CAD build for the part. Positions are in the model's coordinates, mm. Face numbers are marked on the shaded views. A direction names the side the tool comes from. Give positions to 0.01 mm unless a question says otherwise; leave off trailing zeros. Write each loop counter-clockwise with the first axis right and the second up, starting at its lowest first coordinate (ties: lowest second). Pieces come first, ordered by that corner, then holes. Notation, with made-up numbers: (-5.5, 46) - (26.5, 46) arc R21 cw to (26.5, 64) - close; hole circle Ø10 at (71.5, 51). An arc over 180 degrees is marked (long way). Answer as a JSON object with one key per item and string values.
from build123d import *

# Parameters (mm, degrees)
EXTRUDE_1_DEPTH     = 15.1
EXTRUDE_START       = -3.88
EXTRUDE_2_DEPTH     = 3.88
CUT_EXTRUDE_1_REACH = 37.992


with BuildPart() as part:
    # 草图1 → 凸台-拉伸1 (new body)
    with BuildSketch(Plane.XY):
        with BuildLine():
            Line((-15.4, 3.2), (-15.4, 7.25))
            ThreePointArc((-15.4, 7.25), (-14.330939751, 9.830939751), (-11.75, 10.9))
            Line((-11.75, 10.9), (11.75, 10.9))
            ThreePointArc((11.75, 10.9), (14.330939751, 9.830939751), (15.4, 7.25))
            Line((15.4, 7.25), (15.4, -7.25))
            ThreePointArc((15.4, -7.25), (14.330939751, -9.830939751), (11.75, -10.9))
            Line((11.75, -10.9), (3.85, -10.9))
            Line((3.85, -10.9), (-3.85, -10.9))
            Line((-3.85, -10.9), (-11.75, -10.9))
            ThreePointArc((-11.75, -10.9), (-14.330939751, -9.830939751), (-15.4, -7.25))
            Line((-15.4, -7.25), (-15.4, 3.2))
        make_face()
        with BuildLine():
            Line((-13.4, 3.2), (-13.4, 7.25))
            ThreePointArc((-13.4, 7.25), (-12.916726189, 8.416726189), (-11.75, 8.9))
            Line((-11.75, 8.9), (11.75, 8.9))
            ThreePointArc((11.75, 8.9), (12.916726189, 8.416726189), (13.4, 7.25))
            Line((13.4, 7.25), (13.4, -7.25))
            ThreePointArc((13.4, -7.25), (12.916726189, -8.416726189), (11.75, -8.9))
            Line((11.75, -8.9), (3.85, -8.9))
            Line((3.85, -8.9), (-3.85, -8.9))
            Line((-3.85, -8.9), (-11.75, -8.9))
            ThreePointArc((-11.75, -8.9), (-12.916726189, -8.416726189), (-13.4, -7.25))
            Line((-13.4, -7.25), (-13.4, 3.2))
        make_face(mode=Mode.SUBTRACT)
    extrude(amount=-EXTRUDE_1_DEPTH)

    # 草图2 → 凸台-拉伸2 (add)
    with BuildSketch(Plane(origin=(0, 0, -15.1), x_dir=(-1, 0, 0), z_dir=(0, 0, -1)).offset(EXTRUDE_START)):
        with BuildLine():
            Line((-13.4, 6.82), (-13.25, 6.82))
            Line((-13.25, 6.82), (-11.67, 6.82))
            ThreePointArc((-11.67, 6.82), (-11.422512627, 6.922512627), (-11.32, 7.17))
            Line((-11.32, 7.17), (-11.32, 8.75))
            Line((-11.32, 8.75), (-11.32, 8.9))
            Line((-11.32, 8.9), (-11.75, 8.9))
            ThreePointArc((-11.75, 8.9), (-12.916726189, 8.416726189), (-13.4, 7.25))
            Line((-13.4, 7.25), (-13.4, 6.82))
        make_face()
        with BuildLine():
            Line((-13.25, -5.02), (-13.4, -5.02))
            Line((-13.4, -5.02), (-13.4, -7.25))
            ThreePointArc((-13.4, -7.25), (-12.916726189, -8.416726189), (-11.75, -8.9))
            Line((-11.75, -8.9), (-9.52, -8.9))
            Line((-9.52, -8.9), (-9.52, -8.75))
            Line((-9.52, -8.75), (-9.52, -5.87))
            ThreePointArc((-9.52, -5.87), (-9.768959236, -5.268959236), (-10.37, -5.02))
            Line((-10.37, -5.02), (-13.25, -5.02))
        make_face()
        with BuildLine():
            Line((9.52, -8.75), (9.52, -8.9))
            Line((9.52, -8.9), (11.75, -8.9))
            ThreePointArc((11.75, -8.9), (12.916726189, -8.416726189), (13.4, -7.25))
            Line((13.4, -7.25), (13.4, -5.02))
            Line((13.4, -5.02), (13.25, -5.02))
            Line((13.25, -5.02), (10.37, -5.02))
            ThreePointArc((10.37, -5.02), (9.768959236, -5.268959236), (9.52, -5.87))
            Line((9.52, -5.87), (9.52, -8.75))
        make_face()
        with BuildLine():
            Line((11.75, 8.9), (11.32, 8.9))
            Line((11.32, 8.9), (11.32, 8.75))
            Line((11.32, 8.75), (11.32, 7.17))
            ThreePointArc((11.32, 7.17), (11.422512627, 6.922512627), (11.67, 6.82))
            Line((11.67, 6.82), (13.25, 6.82))
            Line((13.25, 6.82), (13.4, 6.82))
            Line((13.4, 6.82), (13.4, 7.25))
            ThreePointArc((13.4, 7.25), (12.916726189, 8.416726189), (11.75, 8.9))
        make_face()
    extrude(amount=EXTRUDE_2_DEPTH)

    # 草图3 → 切除-拉伸1 (cut, up to next)
    with BuildSketch(Plane.ZY.offset(15.4), mode=Mode.PRIVATE) as cut_extrude_1_sk1:
        with BuildLine():
            Line((0.15, 8.9), (-4, 8.9))
            ThreePointArc((-4, 8.9), (-4.247487373, 8.797487373), (-4.35, 8.55))
            Line((-4.35, 8.55), (-4.35, 3.55))
            ThreePointArc((-4.35, 3.55), (-4.247487373, 3.302512627), (-4, 3.2))
            Line((-4, 3.2), (0.15, 3.2))
            Line((0.15, 3.2), (0.15, 8.9))
        make_face()
    cut_extrude_1_tool1 = extrude(cut_extrude_1_sk1.sketch, amount=-CUT_EXTRUDE_1_REACH, mode=Mode.PRIVATE) & part.part
    add(cut_extrude_1_tool1.solids().sort_by_distance((-15.4, 6.05, -2.095539))[0], mode=Mode.SUBTRACT)


solid = part.part
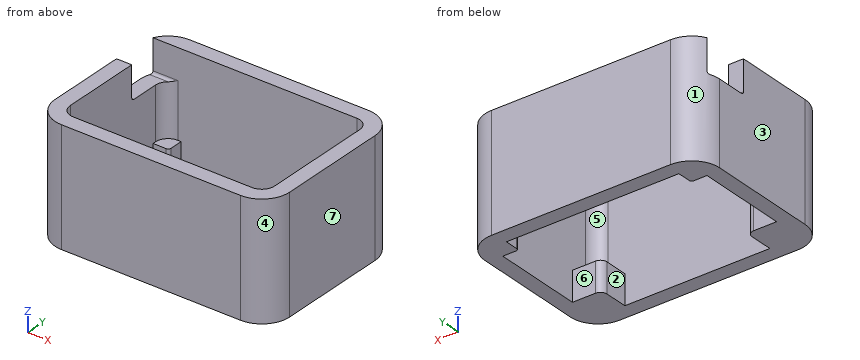
(1) Saw through at D-D, the plane y = -6.5. Give the cut face in (x, z), and give its area (3 significant figures).
Answer key:
{"outline": "(-15.4, -15.1) - (-9.52, -15.1) - (-9.52, -11.22) - (-13.4, -11.22) - (-13.4, 0) - (-15.4, 0) - close; (9.52, -15.1) - (15.4, -15.1) - (15.4, 0) - (13.4, 0) - (13.4, -11.22) - (9.52, -11.22) - close", "area": "90.5 mm²"}
(2) Saw through at A-A, the plane y = -0.25. Give the cut face in (x, z), and give its area (3 significant figures).
Answer key:
{"outline": "(-15.4, -15.1) - (-13.4, -15.1) - (-13.4, 0) - (-15.4, 0) - close; (13.4, -15.1) - (15.4, -15.1) - (15.4, 0) - (13.4, 0) - close", "area": "60.4 mm²"}
(3) Flat gauge pins, fed straight in: P1, Ø0.9, axis at x = -12.5, z = -13, coming from the -Y side; P2, Ø2, axis at x = -15, z = -2.5, coming from the +Y side; P3, Ø1, axis at x = -13, y = 7.5, coming from the +Z side. Where does each tip first touch, or does it go through?
Answer key:
{"P1": "stops at y = -10.89", "P2": "stops at y = 10.12", "P3": "stops at z = -4.35"}
(4) 3-axis set-ups, long thin cutter, end or side, ignore diameter. For the marked faces 5, 6 and 7: which of +Z, -Z, +X, -X, +Y, -Y reach the whole face in a straight line?
Answer key:
{"face 5": "+Z", "face 6": "+Z, -Z", "face 7": "+Z, -Z, +X, +Y, -Y"}
(5) Probe L1, parallel to Y at x = -1, z = -8.25; L2, parallel to X at y = -7, z = -7.5; L3, parallel to Y at x = 11, z = -12. List the from-to ranges inside material, lowest first. Write a range as [from, to].
Answer key:
{"L1": "y = [-10.9, -8.9], [8.9, 10.9]", "L2": "x = [-15.4, -13.4], [13.4, 15.4]", "L3": "y = [-10.9, -5.02], [8.9, 10.9]"}
(6) Saw through at C-C, the plane z = -8.5. Give the cut face in (x, y), and give its area (3 significant figures).
Answer key:
{"outline": "(-15.4, -7.25) arc R3.65 ccw to (-11.75, -10.9) - (11.75, -10.9) arc R3.65 ccw to (15.4, -7.25) - (15.4, 7.25) arc R3.65 ccw to (11.75, 10.9) - (-11.75, 10.9) arc R3.65 ccw to (-15.4, 7.25) - close; hole (-13.4, -7.25) arc R1.65 ccw to (-11.75, -8.9) - (11.75, -8.9) arc R1.65 ccw to (13.4, -7.25) - (13.4, 7.25) arc R1.65 ccw to (11.75, 8.9) - (-11.75, 8.9) arc R1.65 ccw to (-13.4, 7.25) - close", "area": "185 mm²"}
(7) Saw through at B-B, the plane x = 7.5. Give the cut face in (y, z).
Answer key:
{"outline": "(-10.9, -15.1) - (-8.9, -15.1) - (-8.9, 0) - (-10.9, 0) - close; (8.9, -15.1) - (10.9, -15.1) - (10.9, 0) - (8.9, 0) - close"}
(8) Pull direction Y, two halves, no side cores. Call the marked faces 1, 2, 3 and 4: pulls with the +Y half, pulls with the -Y half, needs draft (parallel to the pull), parting line crosses it, or undercut.
Answer key:
{"face 1": "pulls with the +Y half", "face 2": "undercut", "face 3": "needs draft", "face 4": "pulls with the -Y half"}
